The model under review builds one solid part; all positions refer to its coordinate system, in mm. Face numbers are marked on the shaded views. A direction names the side the tool comes from. Give positions to 0.01 mm unless a question says otherwise; leave off trailing zeros. Order: outer loops, then holes, each group sorted by start corner. A loop starts at its lowest first (then second) coordinate and runs counter-clockwise, first axis right, second up. Notation, with made-up numbers: (63.25, 27.25) - (93.25, 27.25) arc R18 cw to (93.25, 58.25) - close; hole circle Ø1 at (42, -29). An arc over 180 degrees is marked (long way). Use CSV: the item, a comma, the result in double quotes. Start each with the question number.
1. To check wall thickness, follow line 1 (Z direction, x = 0, y = 7.25) (3 decimals); line 2 (X direction, y = 33, z = 0.25); line 3 (X direction, y = 4.5, z = -1). State the ranges of each line that lie inside material, in increasing order. Write a range as [from, to].
2. Take a section at B-B, the plane y = 26.5. State the section outline as (x, z) points (3 decimals), then the cut area to 3 significant figures.
3. Take a section at A-A, the plane y = 20.5. State the section outline as (x, z) points (3 decimals).
4. Machinability: for the marked faces 1 and 2, which of the approach directions +Z, -Z, +X, -X, +Y, -Y give a long, thin tool a straight path to every point of the face, cutting with its end or side? Answer none if there is none.
5. Draft analysis for pull direction X (two halves, no side actions). For the marked faces 3, 4 and 5, state which applies: released by +X, released by -X, zero draft, split by the parting line, or undercut.
6. For pin 1 (1 mm diameter, centred on x = 2, y = 25, fed in from +Z); pin 2 (2 mm diameter, centred on x = 0, z = -2, fed in from -Y); pin 3 (1 mm diameter, centred on x = 2, y = 14.5, fed in from -Z); pin 4 (2 mm diameter, centred on x = 0, z = 0, fed in from -Y), all flat-tipped, find the tip position at first contact; note any pin that passes through.
7. Take a section at D-D, the plane x = -2. State the section outline as (y, z) points (3 decimals), then the cut area to 3 significant figures.
8. Take a section at C-C, the plane z = -1.75. State the section outline as (x, y) points (3 decimals), then the cut area to 3 significant figures.
```python
from build123d import *

# Parameters (mm, degrees)
SKETCH1_R                 = 3.175
BOSS_EXTRUDE1_DEPTH       = 34.925
M3X0_5_TAPPED_HOLE1_D     = 2.5
M3X0_5_TAPPED_HOLE1_DEPTH = 12.7
M3X0_5_TAPPED_HOLE1_TIP   = 0.751075774
M3X0_5_TAPPED_HOLE2_D     = 2.5
M3X0_5_TAPPED_HOLE2_DEPTH = 12.7
M3X0_5_TAPPED_HOLE2_TIP   = 0.751075774


with BuildPart() as part:
    # Sketch1 → Boss-Extrude1 (new body)
    with BuildSketch(Plane(origin=(0, 0, 0), x_dir=(1, 0, 0), z_dir=(0, 1, 0))):
        Circle(SKETCH1_R)
    extrude(amount=BOSS_EXTRUDE1_DEPTH)

    # M3x0.5 Tapped Hole1
    with Locations(Plane(origin=(0, 34.925, 0), x_dir=(1, 0, 0), z_dir=(0, 1, 0))):
        with Locations((0, 0)):
            Hole(M3X0_5_TAPPED_HOLE1_D / 2, depth=M3X0_5_TAPPED_HOLE1_DEPTH)
            with Locations((0, 0, -(M3X0_5_TAPPED_HOLE1_DEPTH + M3X0_5_TAPPED_HOLE1_TIP / 2))):  # 118° drill point
                Cone(0, M3X0_5_TAPPED_HOLE1_D / 2, M3X0_5_TAPPED_HOLE1_TIP, mode=Mode.SUBTRACT)

    # M3x0.5 Tapped Hole2
    with Locations(Plane(origin=(0, 0, 0), x_dir=(-1, 0, 0), z_dir=(0, -1, 0))):
        with Locations((0, 0)):
            Hole(M3X0_5_TAPPED_HOLE2_D / 2, depth=M3X0_5_TAPPED_HOLE2_DEPTH)
            with Locations((0, 0, -(M3X0_5_TAPPED_HOLE2_DEPTH + M3X0_5_TAPPED_HOLE2_TIP / 2))):  # 118° drill point
                Cone(0, M3X0_5_TAPPED_HOLE2_D / 2, M3X0_5_TAPPED_HOLE2_TIP, mode=Mode.SUBTRACT)


solid = part.part
```
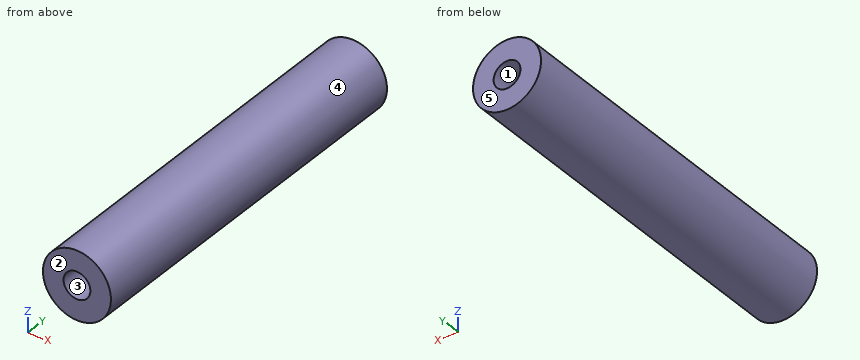
Determined:
1,line 1,"z = [-3.175, -1.25], [1.25, 3.175]"
1,line 2,"x = [-3.17, -1.22], [1.22, 3.17]"
1,line 3,"x = [-3.01, -0.75], [0.75, 3.01]"
2,outline,"circle Ø6.35 at (0, 0); hole circle Ø2.5 at (0, 0)"
2,area,"26.8 mm²"
3,outline,"circle Ø6.35 at (0, 0)"
4,face 1,"+Y"
4,face 2,"+Z, -Z, +X, -X, -Y"
5,face 3,"undercut"
5,face 4,"split by the parting line"
5,face 5,"zero draft"
6,pin 1,"stops at z = 2.8"
6,pin 2,"stops at y = 0"
6,pin 3,"stops at z = -2.8"
6,pin 4,"stops at y = 12.85"
7,outline,"(0, -2.466) - (34.925, -2.466) - (34.925, 2.466) - (0, 2.466) - close"
7,area,"172 mm²"
8,outline,"(-2.649, 0) - (2.649, 0) - (2.649, 34.925) - (-2.649, 34.925) - close"
8,area,"185 mm²"
